Could you check a few things on this model? Use its own coordinates, in mm. A direction names the side the tool comes from. Round coordinates to 2 decimals unless told otherwise and drop trailing zeros. Write each loop counter-clockwise with the first axis right and the second up, starting at its lowest first coordinate (ties: lowest second). Pieces come first, ordered by that corner, then holes. Notation, with made-up numbers: (81, 86) -> (125, 86) arc R7 cw to (125, 94) -> close; hole circle Ø1 at (46, 34.25). An arc over 180 degrees is marked (long way). Return JSON: item names as keys, results as strings.
from build123d import *

# Parameters (mm, degrees)
F1_DEPTH = 7


with BuildPart() as f1:
    # F0 (on Front) → F1 (new body)
    with BuildSketch(Plane.XZ):
        with BuildLine():
            Line((-16, -7.5), (-16, 28.2886903196))
            ThreePointArc((-16, 28.2886903196), (-32.5, 0), (-16, -28.2886903196))
            Line((-16, -28.2886903196), (-16, -7.5))
        make_face()
        with BuildLine():
            Line((16, -7.5), (16, 28.2886903196))
            ThreePointArc((16, 28.2886903196), (0, 32.5), (-16, 28.2886903196))
            Line((-16, 28.2886903196), (-16, -7.5))
            Line((-16, -7.5), (16, -7.5))
        make_face()
        with BuildLine():
            ThreePointArc((16, -28.2886903196), (28.0735640773, -16.3745228938), (32.5, 0))
            ThreePointArc((32.5, 0), (28.0735640773, 16.3745228938), (16, 28.2886903196))
            Line((16, 28.2886903196), (16, -7.5))
            Line((16, -7.5), (16, -28.2886903196))
        make_face()
    extrude(amount=F1_DEPTH)


solid = f1.part
1) I want a section at B-B, the plane y = -4. Please give me the cut outline in (x, z), and give its area (3 significant figures).
Return value:
{"outline": "(-16, -28.29) -> (-16, -7.5) -> (16, -7.5) -> (16, -28.29) arc R32.5 ccw (long way) to start", "area": "2,560 mm²"}
2) If I drill on probe 1 along X at (y, z) = (-0.75, -8); probe 2 along X at (y, z) = (-5, -11.5); probe 3 along Z at (x, y) = (23.5, -4), over which ranges is the centre line in solid material (lowest first)? Write a range as [from, to].
Return value:
{"probe 1": "[-31.5, -16], [16, 31.5]", "probe 2": "[-30.4, -16], [16, 30.4]", "probe 3": "[-22.45, 22.45]"}
3) I want a section at D-D, the plane z = 8.5. Please give me the cut outline in (x, y).
Return value:
{"outline": "(-31.37, -7) -> (31.37, -7) -> (31.37, 0) -> (-31.37, 0) -> close"}
4) I want a section at A-A, the plane z = -9. Please give me the cut outline in (x, y).
Return value:
{"outline": "(-31.23, -7) -> (-16, -7) -> (-16, 0) -> (-31.23, 0) -> close; (16, -7) -> (31.23, -7) -> (31.23, 0) -> (16, 0) -> close"}
5) Will these pins go through, and if not, where does the flat tip stop? pin 1 Ø3 at (x, y) = (-3, -2.5) entering from -Z; pin 2 Ø1 at (y, z) = (-4, 15) entering from +X; pin 3 Ø4 at (x, y) = (-19, -5.5) entering from +Z.
Return value:
{"pin 1": "z = -7.5", "pin 2": "x = 29.09", "pin 3": "z = 27.7"}
6) I want a section at C-C, the plane x = -26. Please give me the cut outline in (y, z).
Return value:
{"outline": "(-7, -19.5) -> (0, -19.5) -> (0, 19.5) -> (-7, 19.5) -> close"}
7) For faces 3 (the face through (-16, -3, -18)), 4 (the face through (0, -7, 9)), which set-ups out of +Z, -Z, +X, -X, +Y, -Y let a thin tool reach every point of the face, with its end or its side?
Return value:
{"face 3": "-Z, +Y, -Y", "face 4": "+Z, -Z, +X, -X, -Y"}
8) Thinking about a two-plate mould opening in X: for faces 1 (the face through (16, -3, -18)), 2 (the face through (0, 0, 9)), which applies, pulls with the +X half, pulls with the -X half, needs draft (parallel to the pull), parting line crosses it, or undercut?
Return value:
{"face 1": "undercut", "face 2": "needs draft"}
